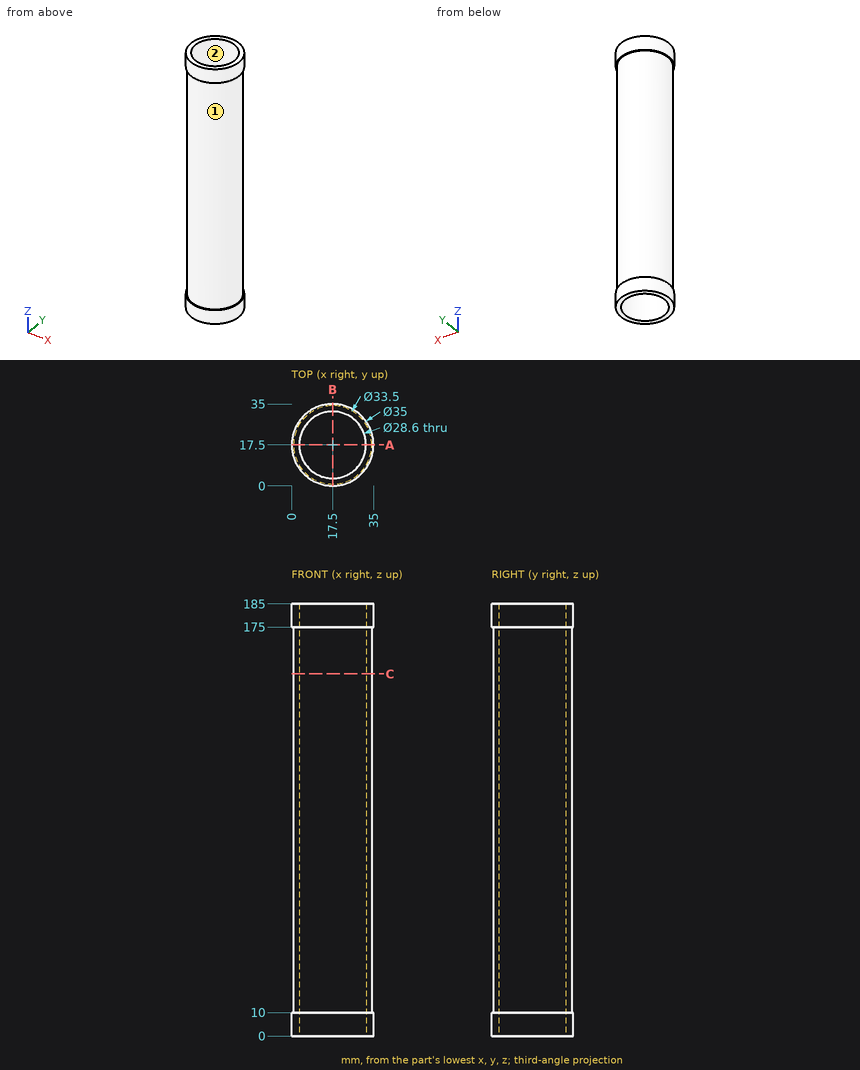
Design review of the part shown in the three views and the two pictorial views. Dimensions are in mm from the part's minimum x, y and z. Round coordinates to 2 decimals unless told otherwise and drop trailing zeros. Loops run counter-clockwise (first coordinate to the right, second up) from the corner with the lowest first, then second, coordinate; pieces in that order, holes last. Notation, with made-up numbers: M -24.75,77 L -19.75,77 A16 ccw -19.75,108 Z; hole C 9,-23 d11. An arc over 180 degrees is marked long. Answer as a JSON object with one key per item and string values.
Item 1: Wall thickness on L1, parallel to Y at x = 17.5, z = 119.5; L2, parallel to X at y = 18, z = 20; L3, parallel to X at y = 19, z = 118.5: over which ranges is each line inside the solid? List them lowest first. Write a range as from..to.
Answer sheet:
{"L1": "y = 0.75..3.2, 31.8..34.25", "L2": "x = 0.76..3.21, 31.79..34.24", "L3": "x = 0.82..3.28, 31.72..34.18"}
Item 2: We need section C-C on z = 155. Give the boundary of the cut face in (x, y).
Answer sheet:
{"outline": "C 17.5,17.5 d33.5; hole C 17.5,17.5 d28.6"}
Item 3: The part is to be moulded in two halves that separate along Z. For the marked faces 1 and 2, say which applies: pulls with the +Z half, pulls with the -Z half, needs draft (parallel to the pull), parting line crosses it, or undercut.
Answer sheet:
{"face 1": "undercut", "face 2": "needs draft"}
Item 4: We need section A-A on y = 17.5. Give the boundary of the cut face in (x, z).
Answer sheet:
{"outline": "M 0,0 L 3.2,0 L 3.2,185 L 0,185 L 0,175 L 0.75,175 L 0.75,10 L 0,10 Z; M 31.8,0 L 35,0 L 35,10 L 34.25,10 L 34.25,175 L 35,175 L 35,185 L 31.8,185 Z"}
Item 5: Clearance check with flat-ended pins moving along their axes: P1, Ø1.5, axis at x = 4, z = 22, coming from the -Y side; P2, Ø2, axis at y = 14.5, z = 58, coming from the +X side; P3, Ø1.5, axis at y = 25.5, z = 27.5, coming from the -X side. State where each tip first meets the part, or that it passes through.
Answer sheet:
{"P1": "stops at y = 6.64", "P2": "stops at x = 34.13", "P3": "stops at x = 2.4"}
